```python
from build123d import *

# Parameters (mm, degrees)
EXTRUDE_2_DEPTH = 35
SKETCH_3_W      = 25.925675676
SKETCH_3_H      = 7
EXTRUDE_3_DEPTH = 1


with BuildPart() as part:
    # 草图2 → 凸台-拉伸2 (new body)
    with BuildSketch(Plane.XY):
        Polygon((-10, 0), (10, 0), (12.962837838, 0), (12.962837838, 7), (9.962837838, 7), (9.962837838, 6), (12, 6), (12, 2), (10, 2), (-10, 2), (-12, 2), (-12, 6), (-9.962837838, 6), (-9.962837838, 7), (-12.962837838, 7), (-12.962837838, 0), align=None)
    extrude(amount=EXTRUDE_2_DEPTH)

    # 草图3 → 凸台-拉伸3 (add)
    with BuildSketch(Plane(origin=(0, 0, 0), x_dir=(-1, 0, 0), z_dir=(0, 0, -1))):
        with Locations((0, 3.5)):
            Rectangle(SKETCH_3_W, SKETCH_3_H)
    extrude(amount=EXTRUDE_3_DEPTH)


solid = part.part
```
Input: part model. Units: mm. Frame: model coordinates. A direction names the side the tool comes from. Give positions to 0.01 mm unless a question says otherwise; leave off trailing zeros. Loops run counter-clockwise (first coordinate to the right, second up) from the corner with the lowest first, then second, coordinate; pieces in that order, holes last. Notation, with made-up numbers: (35, -9.5) -> (47, -9.5) arc R35 cw to (47, 27.5) -> close; hole circle Ø9 at (-40, 40). An arc over 180 degrees is marked (long way). Use a Markdown table: item, result.
Q1. First-contact query: P1, Ø10, axis at x = 4.5, z = 14, coming from the +Y side; P2, Ø4, axis at x = -6, y = 5, coming from the +Z side. Flat tips, straight axial feed; report the tip coordinate or a pass-through.
Entries:
| item | result |
|---|---|
| P1 | stops at y = 2 |
| P2 | stops at z = 0 |
Q2. Section query C-C, the plane x = 5.25. Return the cut outline in (y, z).
Entries:
| item | result |
|---|---|
| outline | (0, -1) -> (7, -1) -> (7, 0) -> (2, 0) -> (2, 35) -> (0, 35) -> close |
Q3. Ray query, probe 1 along X at (y, z) = (5.25, 23); probe 2 along Y at (x, z) = (-10.75, 28); probe 3 along X at (y, z) = (6.25, 22.5). Return the intervals inside material, ascending. Write a range as from..to.
Entries:
| item | result |
|---|---|
| probe 1 | x = -12.96..-12, 12..12.96 |
| probe 2 | y = 0..2, 6..7 |
| probe 3 | x = -12.96..-9.96, 9.96..12.96 |
Q4. Section query A-A, the plane y = 4.25. Return the cut outline in (x, z), plus the area to 3 significant figures.
Entries:
| item | result |
|---|---|
| outline | (-12.96, -1) -> (12.96, -1) -> (12.96, 35) -> (12, 35) -> (12, 0) -> (-12, 0) -> (-12, 35) -> (-12.96, 35) -> close |
| area | 93.3 mm² |
Q5. Access query for faces 4 (the flat face through (11, 6, 17)), 5 (the flat face through (-9.963, 6.5, 17.3)), 6 (the flat face through (11, 7, 14)). Directions: +Z, -Z, +X, -X, +Y, -Y. A direction counts if a zero-diameter tool reaches every point of the face in a straight line with its end or side. Return the directions, or none.
Entries:
| item | result |
|---|---|
| face 4 | +Z |
| face 5 | +Z, +Y |
| face 6 | +Z, -Z, +X, -X, +Y |
Q6. Section query B-B, the plane z = 21.5. Return the cut outline in (x, y).
Entries:
| item | result |
|---|---|
| outline | (-12.96, 0) -> (12.96, 0) -> (12.96, 7) -> (9.96, 7) -> (9.96, 6) -> (12, 6) -> (12, 2) -> (-12, 2) -> (-12, 6) -> (-9.96, 6) -> (-9.96, 7) -> (-12.96, 7) -> close |
Q7. Pull-direction query (X, two-part tool) for faces 1 (the flat face through (12.963, 3, 17)), 2 (the flat face through (0, 0, 17)), 3 (the flat face through (-12, 4, 17)); classes: pulls with the +X half, pulls with the -X half, needs draft (parallel to the pull), parting line crosses it, or undercut.
Entries:
| item | result |
|---|---|
| face 1 | pulls with the +X half |
| face 2 | needs draft |
| face 3 | undercut |
